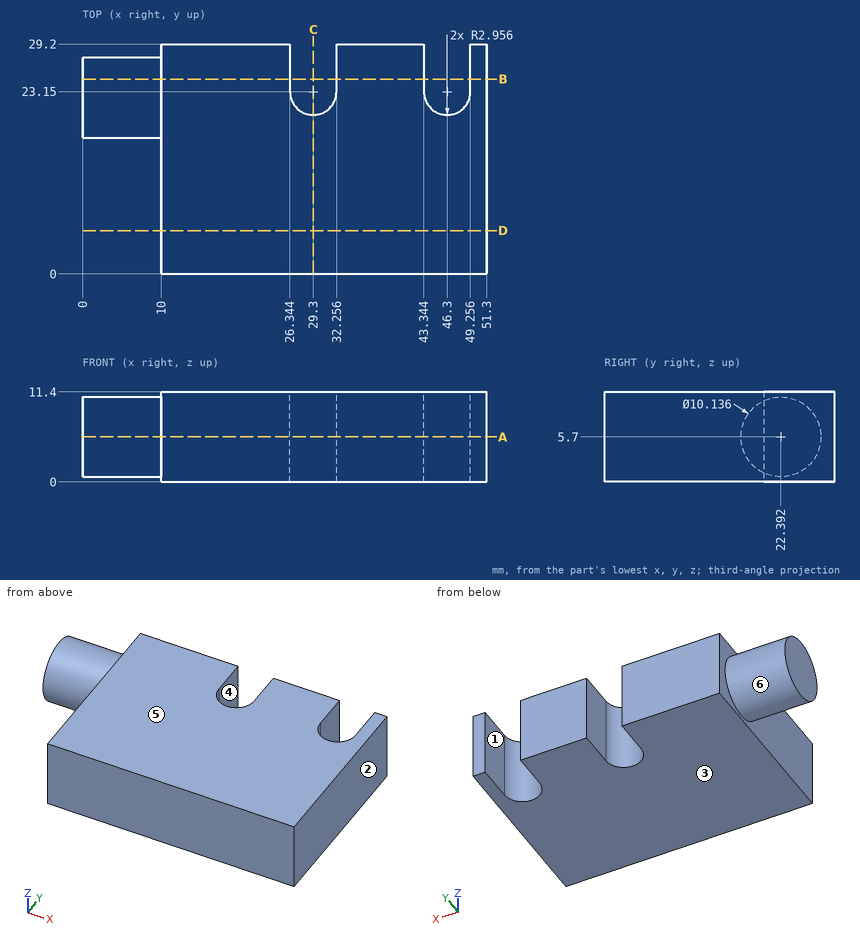
Here's the drawing with two shaded views (mm, measured from the low corner). I have some questions. A direction names the side the tool comes from. Round coordinates to 2 decimals unless told otherwise and drop trailing zeros. Loops run counter-clockwise (first coordinate to the right, second up) from the corner with the lowest first, then second, coordinate; pieces in that order, holes last. Notation, with made-up numbers: (36.25, 71.25) - (57.25, 71.25) arc R35 cw to (57.25, 108.25) - close; hole circle Ø1 at (16, 23). An arc over 180 degrees is marked (long way). Use CSV: the item, a comma, the result in double quotes.
Item 1: Will this pin go through, and if not, where does the flat tip stop? pin 1 (1 mm diameter, centred on y = 6.5, z = 2.5, fed in from -X).
Here are the results:
pin 1,"stops at x = 10"
Item 2: I need wall thicknesses on L1, parallel to X at y = 23, z = 10; L2, parallel to X at y = 26.75, z = 2; L3, parallel to X at y = 7, z = 8.25. Which ranges of each line are inside material? Lowest first, please. Write a range as [from, to].
Here are the results:
L1,"x = [0, 26.35], [32.25, 43.35], [49.25, 51.3]"
L2,"x = [10, 26.34], [32.26, 43.34], [49.26, 51.3]"
L3,"x = [10, 51.3]"
Item 3: For the marked faces 4, 5 and 6, which set-ups out of +Z, -Z, +X, -X, +Y, -Y let a thin tool reach every point of the face, with its end or its side?
Here are the results:
face 4,"+Z, -Z, +Y"
face 5,"+Z, +X, -X, +Y, -Y"
face 6,"-X"
Item 4: If we section it at A-A on z = 5.7: List the corners of the cut face in (x, y) for me, then the cut area to 3 significant figures.
Here are the results:
outline,"(0, 17.32) - (10, 17.32) - (10, 0) - (51.3, 0) - (51.3, 29.2) - (49.26, 29.2) - (49.26, 23.15) arc R2.96 cw to (43.34, 23.15) - (43.34, 29.2) - (32.26, 29.2) - (32.26, 23.15) arc R2.96 cw to (26.34, 23.15) - (26.34, 29.2) - (10, 29.2) - (10, 27.46) - (0, 27.46) - close"
area,"1,210 mm²"
Item 5: If we section it at B-B on y = 24.75: List the corners of the cut face in (x, z) for me, then the cut area to 3 significant figures.
Here are the results:
outline,"(0, 1.21) - (10, 1.21) - (10, 0) - (26.34, 0) - (26.34, 11.4) - (10, 11.4) - (10, 10.19) - (0, 10.19) - close; (32.26, 0) - (43.34, 0) - (43.34, 11.4) - (32.26, 11.4) - close; (49.26, 0) - (51.3, 0) - (51.3, 11.4) - (49.26, 11.4) - close"
area,"426 mm²"
Item 6: If we section it at D-D on y = 5.5: List the corners of the cut face in (x, z) for me, then the cut area to 3 significant figures.
Here are the results:
outline,"(10, 0) - (51.3, 0) - (51.3, 11.4) - (10, 11.4) - close"
area,"471 mm²"
Item 7: If we section it at C-C on x = 29.3: List the corners of the cut face in (y, z) for me.
Here are the results:
outline,"(0, 0) - (20.19, 0) - (20.19, 11.4) - (0, 11.4) - close"
Item 8: If we mould it in two halves opening along X, with no side actions, what happens to the marked faces 1, 2 and 3? For each: pulls with the +X half, pulls with the -X half, needs draft (parallel to the pull), parting line crosses it, or undercut.
Here are the results:
face 1,"undercut"
face 2,"pulls with the +X half"
face 3,"needs draft"
